Input: dimensioned drawing with shaded views. Units: mm. Origin: part minimum x, y, z. Round coordinates to 2 decimals unless told otherwise and drop trailing zeros. Loops run counter-clockwise (first coordinate to the right, second up) from the corner with the lowest first, then second, coordinate; pieces in that order, holes last. Notation, with made-up numbers: (28.25, 88) - (66.25, 88) arc R23 cw to (66.25, 100) - close; hole circle Ø3 at (-35, -2.75). An arc over 180 degrees is marked (long way). One line per question, with ' | ' between items. Start each with the question number.
Item 1: Section C-C, the plane y = 69. Return loops of the section in (x, z) (3 decimals).
Item 2: Section B-B, the plane x = 6.5. Return loops of the section in (y, z) (3 decimals), plus the area to 3 significant figures.
Item 3: Section A-A, the plane z = 29.5. Return loops of the section in (x, y).
Item 4: First-contact query: pin 1 (4 mm diameter, centred on x = 9.5, y = 116, fed in from -Z) (3 decimals). Flat tip, straight axial feed; report the tip coordinate or a pass-through.
Item 5: Material intervals for line 1 along Y through (x, z) = (0.5, 69); line 2 along Z through (x, y) = (7.5, 83) (3 decimals); line 3 along Z through (x, y) = (10.75, 24) (3 decimals), sorted ascending.
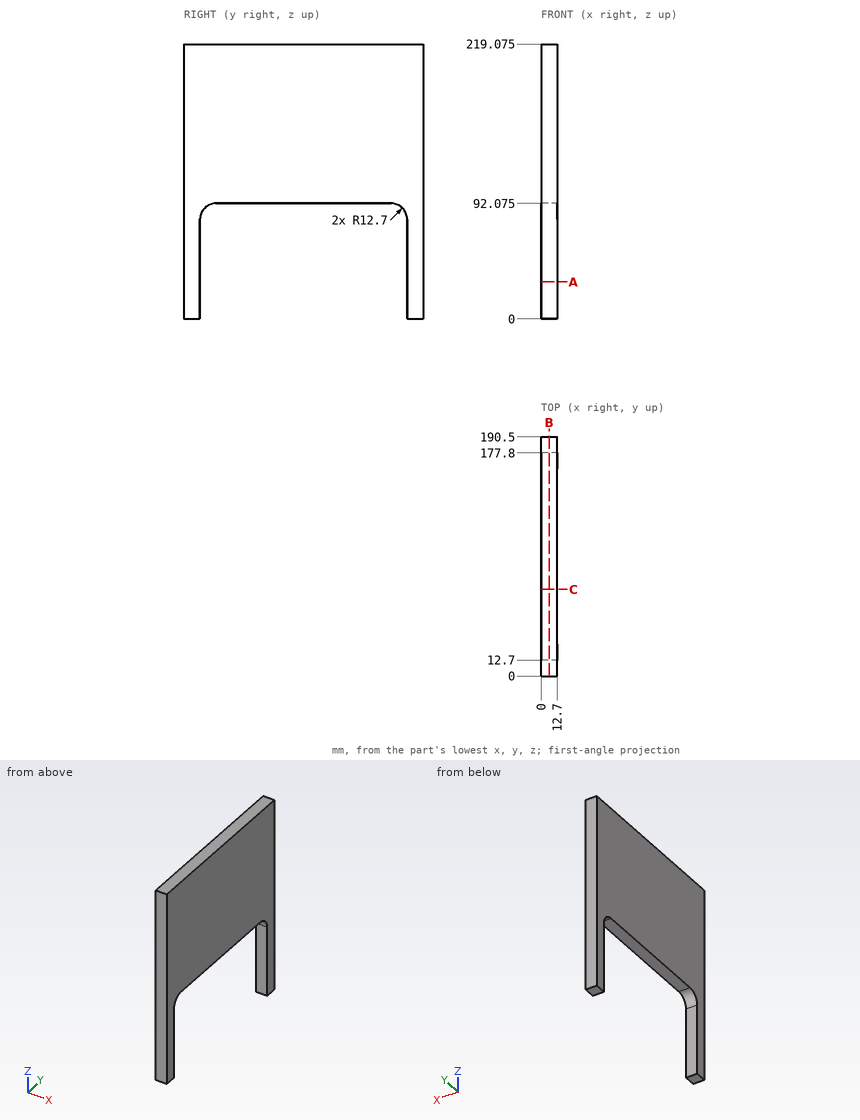
Return value:
1) outline: (0, 92.075) - (12.7, 92.075) - (12.7, 219.075) - (0, 219.075) - close
2) outline: (0, 0) - (12.7, 0) - (12.7, 79.375) arc R12.7 cw to (25.4, 92.075) - (165.1, 92.075) arc R12.7 cw to (177.8, 79.375) - (177.8, 0) - (190.5, 0) - (190.5, 219.075) - (0, 219.075) - close | area: 26,600 mm2
3) outline: (0, 0) - (12.7, 0) - (12.7, 12.7) - (0, 12.7) - close; (0, 177.8) - (12.7, 177.8) - (12.7, 190.5) - (0, 190.5) - close
4) pin 1: z = 92.075
5) line 1: 0 to 12.7, 177.8 to 190.5 | line 2: 92.075 to 219.075 | line 3: 91.998 to 219.075
